from build123d import *

# Parameters (mm, degrees)
F0_R      = 29.7932126591
F1_DEPTH  = 8.382
F2_R      = 24.5943618738
F3_DEPTH  = 38.862
F4_R      = 22.6553491942
F5_DEPTH  = 31.496
F7_DEPTH  = 39.116
F8_R      = 21.4427670818
F9_DEPTH  = 2.286
F10_DEPTH = 25.4


with BuildPart() as f1:
    # F0 (on Front) → F1 (new body)
    with BuildSketch(Plane.XZ):
        with Locations((-5.3459531628, 3.9943419397)):
            Circle(F0_R)
    extrude(amount=F1_DEPTH)

    # F2 (on face) → F3 (join)
    with BuildSketch(Plane.XZ.offset(8.382)):
        with Locations((-5.3459531628, 3.9943419397)):
            Circle(F2_R)
    extrude(amount=F3_DEPTH)

    # F4 (on face) → F5 (join)
    with BuildSketch(Plane.XZ.offset(47.244)):
        with Locations((-5.3459531628, 3.9943419397)):
            Circle(F4_R)
    extrude(amount=F5_DEPTH)

    # F6 (on face) → F7 (cut)
    with BuildSketch(Plane.XZ.offset(47.244)):
        with BuildLine():
            Line((-18.2745195925, -16.927770909), (-18.2745195925, -15.7896652818))
            Line((-18.2745195925, -15.7896652818), (-18.9284321236, -16.5092894767))
            ThreePointArc((-18.9284321236, -16.5092894767), (-18.6031272056, -16.7211105627), (-18.2745195925, -16.927770909))
        make_face()
    extrude(amount=-F7_DEPTH, mode=Mode.SUBTRACT)

    # F8 (on face) → F9 (cut)
    with BuildSketch(Plane(origin=(0, 0, 0), x_dir=(-1, 0, 0), z_dir=(0, 1, 0))):
        with Locations((5.3459531628, 3.9943419397)):
            Circle(F8_R)
    extrude(amount=-F9_DEPTH, mode=Mode.SUBTRACT)

    # F10 (cut): a face of the model
    f10_faces = [f1.faces().sort_by_distance(p)[0] for p in [
        (-5.3459531628, -2.286, 3.9943419397),
    ]]
    extrude(f10_faces, amount=-F10_DEPTH, mode=Mode.SUBTRACT)


solid = f1.part
Part model, mm, in its own coordinate system. A direction names the side the tool comes from. Coordinates: 2 decimals unless noted, no trailing zeros. Write each loop counter-clockwise with the first axis right and the second up, starting at its lowest first coordinate (ties: lowest second). Pieces come first, ordered by that corner, then holes. Notation, with made-up numbers: M 23,54 L 60,54 A28 ccw 60,72 Z; hole C 24,-5.75 d3. An arc over 180 degrees is marked long. Return JSON: item names as keys, results as strings.
1. 3-axis set-ups, long thin cutter, end or side, ignore diameter. For faces 4 (the face through (11.67, -13.649, -9.053)), 5 (the face through (-23.324, -62.772, -9.791)), 6 (the face through (-6, -78.74, 4)): which of +Z, -Z, +X, -X, +Y, -Y reach the whole face in a straight line?
Determined:
{"face 4": "+Y", "face 5": "-Y", "face 6": "+Z, -Z, +X, -X, -Y"}
2. Saw through at B-B, the plane z = 20. Write the cut outline in (x, y), then the cut area to 3 significant figures.
Determined:
{"outline": "M -30.47,-8.38 L -24.02,-8.38 L -24.02,-47.24 L -21.38,-47.24 L -21.38,-78.74 L 10.69,-78.74 L 10.69,-47.24 L 13.33,-47.24 L 13.33,-8.38 L 19.78,-8.38 L 19.78,0 L 8.92,0 L 8.92,-27.69 L -19.62,-27.69 L -19.62,0 L -30.47,0 Z", "area": "2,090 mm²"}
3. Pull direction Z, two halves, no side cores. Call faces 1 (the face through (-5, -27.686, 4)), 2 (the face through (-11.8, -4.13, -25.09)), 3 (the face through (-26, 0, 11)): pulls with the +Z half, pulls with the -Z half, needs draft (parallel to the pull), parting line crosses it, or undercut.
Determined:
{"face 1": "undercut", "face 2": "parting line crosses it", "face 3": "needs draft"}
4. Probe L1, parallel to Y at x = -21.5, z = -10; L2, parallel to Z at x = -8, y = -26.5; L3, parallel to Y at x = 13, z = -13.5. List the from-to ranges inside material, lowest first.
Determined:
{"L1": "-78.74 to -27.69", "L2": "-20.46 to -17.28, 25.27 to 28.45", "L3": "-8.38 to 0"}
5. Flat gauge pins, fed straight in: pin 1 Ø4 at (y, z) = (-13.5, 23) entering from -X; pin 2 Ø6 at (y, z) = (-36.5, 14) entering from +X; pin 3 Ø12 at (x, y) = (15.5, -46.5) entering from -Z. Where does each tip first touch, or does it go through?
Determined:
{"pin 1": "x = -23.11", "pin 2": "x = 18.23", "pin 3": "z = -15.61"}
6. Saw through at A-A, the plane x = 0. Write the cut outline in (y, z), then the cut area to 3 significant figures.
Determined:
{"outline": "M -78.74,-18.02 L -47.24,-18.02 L -47.24,-20.01 L -8.38,-20.01 L -8.38,-25.32 L 0,-25.32 L 0,-16.77 L -27.69,-16.77 L -27.69,24.76 L 0,24.76 L 0,33.3 L -8.38,33.3 L -8.38,28 L -47.24,28 L -47.24,26.01 L -78.74,26.01 Z", "area": "2,590 mm²"}
7. Saw through at C-C, the plane y = -20. Write the cut outline in (x, z), then the cut area to 3 significant figures.
Determined:
{"outline": "M -18.93,-16.51 L -18.27,-15.79 L -18.27,-16.93 A24.59 ccw long Z; hole C -5.35,3.99 d42.89", "area": "455 mm²"}
8. Saw through at D-D, the plane y = -45.5. Write the cut outline in (x, z), then the cut area to 3 significant figures.
Determined:
{"outline": "M -18.93,-16.51 L -18.27,-15.79 L -18.27,-16.93 A24.59 ccw long Z", "area": "1,900 mm²"}
